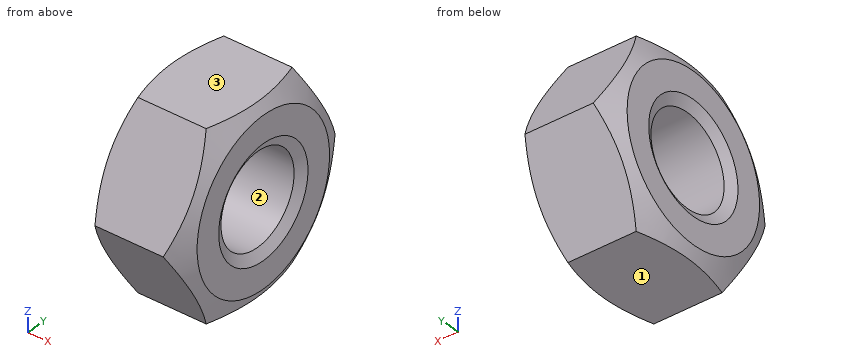
Autodesk Inventor part; units mm, degrees
ref_plane "Work Plane1" through (-10.9812, 0, 0) normal (0, -0.8660254, -0.5) x (1, 0, 0)
ref_plane "YZ Plane" through (0, 0, 0) normal (1, 0, 0) x (0, 1, 0)
ref_plane "XZ Plane" through (0, 0, 0) normal (0, 1, 0) x (-1, 0, 0)
sketch "Szkic1" plane through (0, 0, 0) normal (1, 0, 0) x (0, 1, 0)
  line L0 (-5.7735, 0) -> (-2.8868, 5)
  line L1 (-2.8868, 5) -> (2.8868, 5)
  line L2 (2.8868, 5) -> (5.7735, 0)
  line L3 (5.7735, 0) -> (2.8868, -5)
  line L4 (2.8868, -5) -> (-2.8868, -5)
  line L5 (-2.8868, -5) -> (-5.7735, 0)
  point P0 (0, 0)
  point P1 (0, 0)
  dimension "d0" = 11.547
extrude "Bryła" add sketch "Szkic1" along normal blind 5.2
sketch "Szkic2" plane through (0, 0, 0) normal (0, 0, 1) x (1, 0, 0)
  line L0 (0, 2.8868) -> (0, 5.7735)
  line L1 (0, 5.7735) -> (5.2, 5.7735)
  line L2 (5.2, 2.8868) -> (5.2, 5.7735)
  line L3 (-1.04, 0) -> (6.24, 0)
  line L4 (0.7641, 5.7735) -> (0, 4.45)
  line L5 (4.4359, 5.7735) -> (5.2, 4.45)
  dimension "d3" = 30
  dimension "d4" = 30
  dimension "d5" = 8.9
  dimension "d6" = 8.9
revolve "Faza1" cut sketch "Szkic2" angle 360 about axis through (-10, 0, 0) along (1, 0, 0)
sketch "Szkic3" plane through (5.2, 0, 0) normal (1, 0, 0) x (0, 0, -1)
  arc A0 (-0.625, -1.0825) -> (0.625, -1.0825) centre (0, 0) ccw
hole "Gwint" at (5.2, 0, 0) direction (-1, 0, 0) diameter 4.917 end through all
chamfer "Faza2" distance 0.5413 angle 30 1 edges at (5.2, 0, 2.4585) measured on face at (5.2, 3.7371, -0.4538)
chamfer "Faza3" distance 0.5413 angle 30 1 edges at (0, 0, 2.4585) measured on face at (0, 3.7371, -0.4538)
ref_plane "Work Plane1" through (-10.9812, 0, 0) normal (0, -0.8660254, -0.5) x (1, 0, 0)
equation "\"d0\" = 1.1547 * SW"
equation "\"d1\" = KOH"
equation "\"d8\" = -0.5 * GD1 + 0.5 * NND"
equation "\"d40\" = -0.5 * GD1 + 0.5 * NND"
equation "\"d10\" = -0.5 * GD1 + 0.5 * NND"
equation "\"d41\" = -0.5 * GD1 + 0.5 * NND"
equation "\"d3\" = ANG1"
equation "\"d4\" = ANG2"
equation "\"d5\" = SW0"
equation "\"d6\" = SW01"
equation "\"ANG1\" = 30deg"
equation "\"ANG2\" = 30deg"
equation "\"NND\" = 6"
equation "\"KOH\" = 5.2"
equation "\"SW0\" = 8.9"
equation "\"SW01\" = 8.9"
equation "\"GUL\" = 0.541266 * PTC"
equation "\"THREADDIA\" = 6"
equation "\"TOA\" = 30deg"
equation "\"PTC\" = 1"
equation "\"E0\" = 1.155 * SW"
equation "\"GAL\" = 0.541266 * PTC"
properties part number "ISO 4032 - M6" material "Stal nierdzewna 440C"
CAD build for the part. Positions are in the model's coordinates, mm. Face numbers are marked on the shaded views. Round coordinates to 2 decimals unless told otherwise and drop trailing zeros. Order: outer loops, then holes, each group sorted by start corner. A loop starts at its lowest first (then second) coordinate and runs counter-clockwise, first axis right, second up.
Item 1: Saw through at A-A on y = 0. Write the cut outline in (x, z), then the cut area to 3 significant figures.
Item 2: Mould opens along Z. For the marked faces 1, 2 and 3 say: pulls with the +Z half, pulls with the -Z half, needs draft (parallel to the pull), parting line crosses it, or undercut.
Item 3: Saw through at B-B on x = 3.7. Write the cut outline in (y, z), then the cut area to 3 significant figures.
Item 4: Pin check, flat tips, straight feed: pin 1 (2 mm diameter, centred on x = 1, z = -3, fed in from -Y); pin 2 (4.5 mm diameter, centred on y = 0, z = 0, fed in from -X); pin 3 (6 mm diameter, centred on y = 4.5, z = -4, fed in from -X). Stop position of each tip, or through.
Item 5: Probe line 1 along Z through (x, y) = (3.1, 0); line 2 along Y through (x, z) = (0.65, -1.5); line 3 along Z through (x, y) = (0.4, 0.25). List the from-to ranges inside material, lowest first.
Reported:
1. outline: (0, -4.45) - (0.32, -5) - (4.88, -5) - (5.2, -4.45) - (5.2, -3) - (4.89, -2.46) - (0.31, -2.46) - (0, -3) - close; (0, 3) - (0.31, 2.46) - (4.89, 2.46) - (5.2, 3) - (5.2, 4.45) - (4.88, 5) - (0.32, 5) - (0, 4.45) - close
1. area: 25.7 mm2
2. face 1: pulls with the -Z half
2. face 2: undercut
2. face 3: pulls with the +Z half
3. outline: (-5.77, 0) - (-2.89, -5) - (2.89, -5) - (5.77, 0) - (2.89, 5) - (-2.89, 5) - close; hole circle Ø4.92 at (0, 0)
3. area: 67.6 mm2
4. pin 1: stops at y = -4.62
4. pin 2: passes through
4. pin 3: stops at x = 0
5. line 1: z = -5 to -2.46, 2.46 to 5
5. line 2: y = -4.91 to -1.95, 1.95 to 4.91
5. line 3: z = -5 to -2.45, 2.45 to 5
